Build history of the part. All positions in model axes, mm. Round coordinates to 2 decimals unless told otherwise and drop trailing zeros. Write each loop counter-clockwise with the first axis right and the second up, starting at its lowest first coordinate (ties: lowest second). Pieces come first, ordered by that corner, then holes.
1) Flat gauge pins, fed straight in: pin 1 (0.6 mm diameter, centred on x = 84, y = -1, fed in from +Z); pin 2 (0.6 mm diameter, centred on y = -1.5, z = 59.5, fed in from +X). Where does each tip first touch, or does it go through?
2) Saw through at C-C (x = 157). Write the cut outline in (y, z), plus the area to 3 significant figures.
3) Saw through at A-A (z = 62). Write the cut outline in (x, y).
4) Wall check: probe 1 along Z at (x, y) = (131, -0.4); probe 2 along Z at (x, y) = (139, -0.75); probe 3 along X at (y, z) = (-1.4, 17). Give the ranges that are in metal, low to high.
5) Saw through at D-D (z = 84). Write the cut outline in (x, y).
6) Saw through at B-B (y = -0.7). Write the cut outline in (x, z).
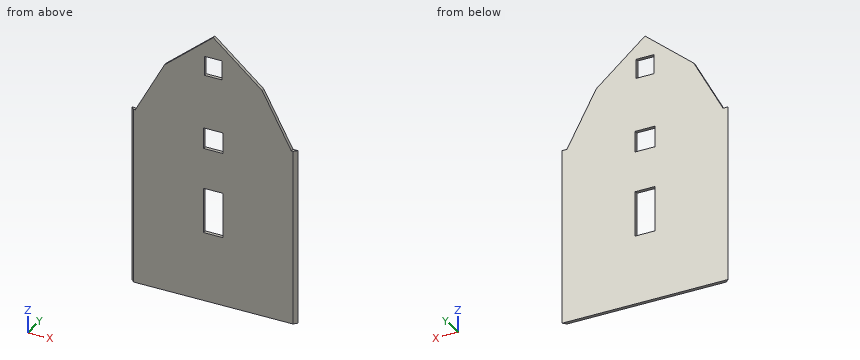
from build123d import *

# Parameters (mm, degrees)
F0_W     = 12
F0_H     = 28
F1_DEPTH = 2
F3_DEPTH = 250
F5_DEPTH = 250


with BuildPart() as f1:
    # F0 (on Front) → F1 (new body)
    with BuildSketch(Plane.XZ):
        Polygon((85.290909, -39.870985), (133.290909, -39.870985), (184.290909, -39.870985), (184.290909, -11.236302), (184.290909, 69.079015), (181.290909, 69.079015), (163.290909, 102.380682), (133.290909, 127.629015), (103.290909, 102.380682), (85.290909, 69.079015), (82.290909, 69.079015), (82.290909, -39.870985), align=None)
        with Locations((133.290909, 16.979015)):
            Rectangle(F0_W, F0_H, mode=Mode.SUBTRACT)
        Polygon((133.290909, 69.079015), (139.290909, 69.079015), (139.290909, 56.079015), (127.290909, 56.079015), (127.290909, 69.079015), align=None, mode=Mode.SUBTRACT)
        Polygon((138.790909, 114.380682), (138.790909, 102.380682), (133.290909, 102.380682), (127.790909, 102.380682), (127.790909, 114.380682), align=None, mode=Mode.SUBTRACT)
    extrude(amount=F1_DEPTH)

    # F2 (on face) → F3 (cut)
    with BuildSketch(Plane.XY.offset(69.079015)):
        Polygon((182.290909, -2), (184.290909, -2), (184.290909, 0), align=None)
    extrude(amount=-F3_DEPTH, mode=Mode.SUBTRACT)

    # F4 (on face) → F5 (cut)
    with BuildSketch(Plane.XY.offset(69.079015)):
        Polygon((82.290909, 0), (82.290909, -2), (84.290909, -2), align=None)
    extrude(amount=-F5_DEPTH, mode=Mode.SUBTRACT)


solid = f1.part
Evaluation:
1. pin 1: stops at z = 69.08
1. pin 2: stops at x = 183.09
2. outline: (-2, -39.87) - (0, -39.87) - (0, 107.68) - (-2, 107.68) - close
2. area: 295 mm2
3. outline: (82.29, 0) - (84.29, -2) - (127.29, -2) - (127.29, 0) - close; (139.29, -2) - (182.29, -2) - (184.29, 0) - (139.29, 0) - close
4. probe 1: z = -39.87 to 2.98, 30.98 to 56.08, 69.08 to 102.38, 114.38 to 125.7
4. probe 2: z = -39.87 to 2.98, 30.98 to 56.08, 69.08 to 122.82
4. probe 3: x = 83.69 to 127.29, 139.29 to 182.89
5. outline: (93.36, -2) - (173.23, -2) - (173.23, 0) - (93.36, 0) - close
6. outline: (82.99, -39.87) - (183.59, -39.87) - (183.59, 69.08) - (181.29, 69.08) - (163.29, 102.38) - (133.29, 127.63) - (103.29, 102.38) - (85.29, 69.08) - (82.99, 69.08) - close; hole (127.29, 2.98) - (139.29, 2.98) - (139.29, 30.98) - (127.29, 30.98) - close; hole (127.29, 56.08) - (139.29, 56.08) - (139.29, 69.08) - (127.29, 69.08) - close; hole (127.79, 102.38) - (138.79, 102.38) - (138.79, 114.38) - (127.79, 114.38) - close
